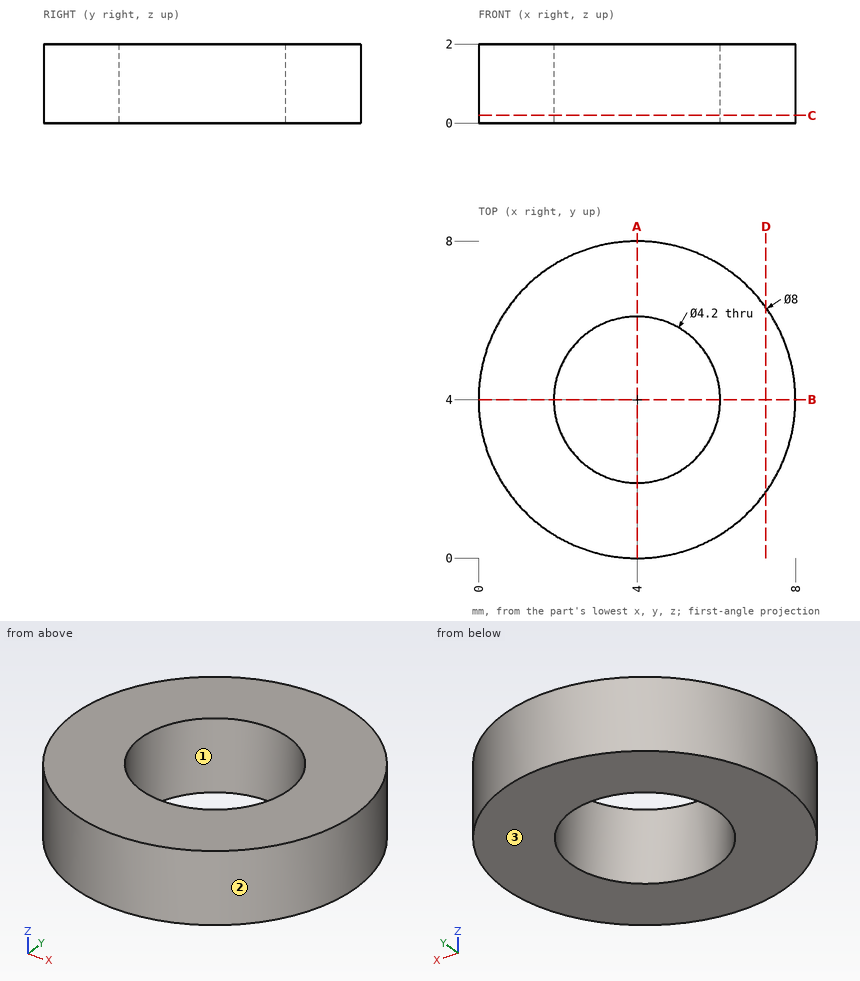
Part print with two shaded views. Sizes in mm from the minimum x, y, z corner. Round coordinates to 2 decimals unless told otherwise and drop trailing zeros. Order: outer loops, then holes, each group sorted by start corner. A loop starts at its lowest first (then second) coordinate and runs counter-clockwise, first axis right, second up. Notation, with made-up numbers: (45, -23) - (74, -23) arc R22 cw to (74, 8) - close; hole circle Ø11 at (-27.75, 80). An arc over 180 degrees is marked (long way). Answer in a Markdown table with one row per item. Add a question column.
(1) Band-saw the part on A-A on x = 4. List the corners of the cut face in (y, z), and give its area (3 significant figures).
(2) Probe L1, parallel to Y at x = 4, z = 1; L2, parallel to Y at x = 5, z = 0.6; L3, parallel to X at y = 5.75, z = 1.35. List the from-to ranges inside material, lowest first. Write a range as [from, to].
(3) Drop flat-ended pins along their axis: pin 1 Ø1 at (y, z) = (2, 1) entering from +X; pin 2 Ø1 at (x, z) = (2, 0.5) entering from +Y. Give the stop position or say it passes through.
(4) Band-saw the part on C-C on z = 0.2. List the corners of the cut face in (x, y), and give its area (3 significant figures).
(5) Mould opens along Y. For the marked faces 1, 2 and 3 say: +Y half, -Y half, draft (parallel to the pull), parting line (faces both ways), or undercut.
(6) Band-saw the part on D-D on x = 7.25. List the corners of the cut face in (y, z), and give its area (3 significant figures).
Data:
| question | item | result |
|---|---|---|
| 1 | outline | (0, 0) - (1.9, 0) - (1.9, 2) - (0, 2) - close; (6.1, 0) - (8, 0) - (8, 2) - (6.1, 2) - close |
| 1 | area | 7.60 mm^2 |
| 2 | L1 | y = [0, 1.9], [6.1, 8] |
| 2 | L2 | y = [0.13, 2.15], [5.85, 7.87] |
| 2 | L3 | x = [0.4, 2.84], [5.16, 7.6] |
| 3 | pin 1 | stops at x = 7.71 |
| 3 | pin 2 | stops at y = 7.71 |
| 4 | outline | circle Ø8 at (4, 4); hole circle Ø4.2 at (4, 4) |
| 4 | area | 36.4 mm^2 |
| 5 | face 1 | undercut |
| 5 | face 2 | parting line |
| 5 | face 3 | draft |
| 6 | outline | (1.67, 0) - (6.33, 0) - (6.33, 2) - (1.67, 2) - close |
| 6 | area | 9.33 mm^2 |
